The figure shows three views and two pictorial views of one solid part (mm, origin at its lowest corner). Answer the questions. A direction names the side the tool comes from. Give positions to 0.01 mm unless a question says otherwise; leave off trailing zeros. Order: outer loops, then holes, each group sorted by start corner. A loop starts at its lowest first (then second) coordinate and runs counter-clockwise, first axis right, second up. Notation, with made-up numbers: M 6,76.25 L 24,76.25 A29 cw 24,99.25 Z; hole C 64,8 d11. An arc over 180 degrees is marked long. One line per item, written item: value.
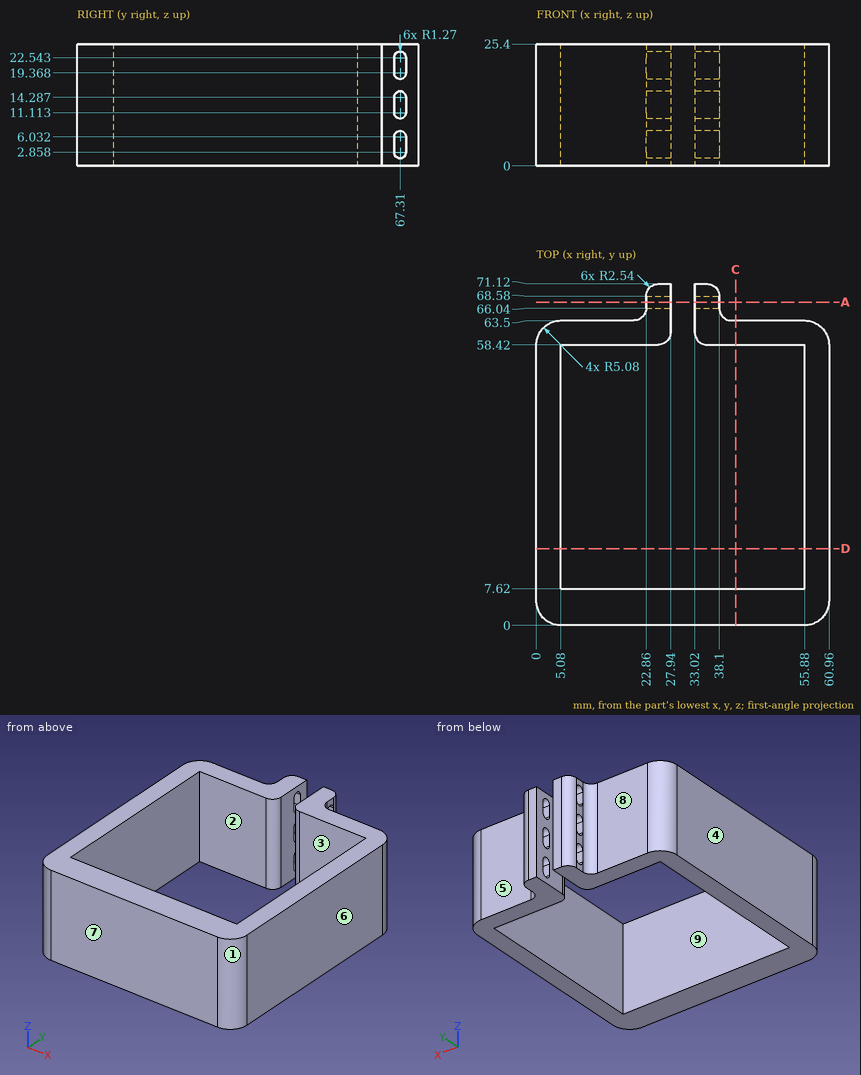
1) Determine the mould class of the marked faces 1, 2, 3 and 4 for opening direction X: +X half, -X half, draft (parallel to the pull), parting line (faces both ways), or undercut.
Reported:
face 1: +X half
face 2: undercut
face 3: undercut
face 4: -X half
2) Find section D-D, the plane y = 16. Write down the section's boundary in (x, z), plus the area to 3 significant figures.
Reported:
outline: M 0,0 L 5.08,0 L 5.08,25.4 L 0,25.4 Z; M 55.88,0 L 60.96,0 L 60.96,25.4 L 55.88,25.4 Z
area: 258 mm^2
3) Find section A-A, the plane y = 67.31. Count the separate pieces of the cut face and the enclosed holes in it.
Reported:
separate pieces: 8
enclosed holes: 0
4) Which of the six approach directions +Z, -Z, +X, -X, +Y, -Y give full straight-line access (tool end or side, diameter ignored) to the marked faces 5, 6, 7, 8 and 9?
Reported:
face 5: +Z, -Z, +X, +Y
face 6: +Z, -Z, +X, +Y, -Y
face 7: +Z, -Z, +X, -X, -Y
face 8: +Z, -Z, -X, +Y
face 9: +Z, -Z
5) Each of these flat-tipped pins is pushed along its axis until it touches: pin 1 Ø5 at (y, z) = (64.5, 9.5) entering from -X (1 decimal); pin 2 Ø1.3 at (y, z) = (67, 16) entering from -X; pin 3 Ø0.8 at (y, z) = (67.5, 24) entering from +X. Where does it stop, or does it pass through?
Reported:
pin 1: stops at x = 1.5
pin 2: stops at x = 22.86
pin 3: stops at x = 38.1
6) Consider probe 1 along X at (y, z) = (55.5, 12.75); probe 2 along Y at (x, z) = (17, 13); probe 3 along Y at (x, z) = (24.5, 4.5) (1 decimal). Determine where each line is inside the solid, lowest interval first.
Reported:
probe 1: x = 0 to 5.08, 55.88 to 60.96
probe 2: y = 0 to 7.62, 58.42 to 63.5
probe 3: y = 0 to 7.6, 58.4 to 66, 68.6 to 71
7) Find section C-C, the plane x = 41.5. Write down the section's boundary in (y, z).
Reported:
outline: M 0,0 L 7.62,0 L 7.62,25.4 L 0,25.4 Z; M 58.42,0 L 63.5,0 L 63.5,25.4 L 58.42,25.4 Z
